Autodesk Inventor part; units mm, degrees
ref_plane "YZ Plane" through (0, 0, 0) normal (1, 0, 0) x (0, 1, 0)
ref_plane "XZ Plane" through (0, 0, 0) normal (0, 1, 0) x (-1, 0, 0)
ref_plane "XY Plane" through (0, 0, 0) normal (0, 0, 1) x (1, 0, 0)
sketch "Sketch1" plane through (0, 0, 0) normal (0, 1, 0) x (-1, 0, 0)
  line L0 (28, 0) -> (-28, 0)
  line L1 (0, -44.1) -> (0, 44.1)
  line L2 (-20, 31.5) -> (20, 31.5)
  line L3 (20, 31.5) -> (20, -31.5)
  line L4 (20, -31.5) -> (-20, -31.5)
  line L5 (-20, -31.5) -> (-20, 31.5)
  line L6 (-20, 31.5) -> (20, -31.5) construction
  line L7 (20, 31.5) -> (-20, -31.5) construction
  point P0 (0, 0)
  dimension "d0" = 40
  dimension "d1" = 63
extrude "Extrusion1" add sketch "Sketch1" along normal blind 20
sketch "Sketch2" plane through (0, 20, 0) normal (0, 1, 0) x (1, 0, 0)
  line L0 (20, 31.5) -> (-20, 31.5)
  line L1 (-20, 31.5) -> (-20, -31.5)
  line L2 (2.8, 26.5) -> (12.8, 26.5)
  line L3 (12.8, 26.5) -> (12.8, -26.5)
  line L4 (12.8, -26.5) -> (2.8, -26.5)
  line L5 (2.8, -26.5) -> (2.8, 26.5)
  line L6 (20, -31.5) -> (20, 31.5)
  dimension "d9" = 10
  dimension "d10" = 53
  dimension "d11" = 5
  dimension "d23" = 7.2
extrude "Extrusion2" cut sketch "Sketch2" against normal blind 11
sketch "Sketch3" plane through (0, 9, 0) normal (0, 1, 0) x (1, 0, 0)
  line L0 (20, -31.5) -> (20, 31.5)
  line L1 (12.8, 26.5) -> (12.8, -26.5)
  line L2 (20, 31.5) -> (-20, 31.5)
  point P0 (0, 0)
  point P1 (7.8, 14.41)
  point P2 (7.8, -14.3)
  dimension "d22" = 5
  dimension "d27" = 17.09
  dimension "d40" = 28.71
  dimension "d41" = 12.2
hole "Hole1" at (7.8, 9, -14.41) at (7.8, 9, 14.3) direction (0, -1, 0) diameter 3.242 end through all
sketch "Sketch5" plane through (0, 9, 0) normal (0, 1, 0) x (1, 0, 0)
  circle A0 centre (7.8, 14.41) radius 1.621
  line L0 (9.8207, 10.91) -> (5.7793, 10.91)
  line L1 (5.7793, 10.91) -> (3.7585, 14.41)
  line L2 (3.7585, 14.41) -> (5.7793, 17.91)
  line L3 (5.7793, 17.91) -> (9.8207, 17.91)
  line L4 (9.8207, 17.91) -> (11.8415, 14.41)
  line L5 (11.8415, 14.41) -> (9.8207, 10.91)
  line L6 (2.8, 26.5) -> (12.8, 26.5)
  line L7 (12.8, -26.5) -> (2.8, -26.5)
  circle A1 centre (7.8, -14.3) radius 1.621
  line L8 (9.8207, -17.8) -> (5.7793, -17.8)
  line L9 (5.7793, -17.8) -> (3.7585, -14.3)
  line L10 (3.7585, -14.3) -> (5.7793, -10.8)
  line L11 (5.7793, -10.8) -> (9.8207, -10.8)
  line L12 (9.8207, -10.8) -> (11.8415, -14.3)
  line L13 (11.8415, -14.3) -> (9.8207, -17.8)
  point P0 (0, 0)
  dimension "d37" = 7
  dimension "d42" = 7
extrude "Extrusion3" cut sketch "Sketch5" against normal blind 4 contours L0 L1 L2 L3 L4 L5 | A1 | L8 L9 L10 L11 L12 L13
sketch "Sketch9" plane through (-20, 0, 31.5) normal (0, 0, 1) x (1, 0, 0)
  line L0 (30.47, 20) -> (30.47, 10)
  line L1 (30.47, 10) -> (-4.63, 10)
  line L2 (-4.63, 10) -> (-4.63, 20)
  line L3 (0, 0) -> (0, 20)
  line L4 (40, 20) -> (0, 20)
  arc A0 (5.8, 20) -> (20.2, 20) centre (13, 20) ccw
  line L5 (-4.63, 20) -> (5.8, 20)
  line L6 (20.2, 20) -> (30.47, 20)
  line L7 (40, 0) -> (40, 20)
  line L8 (5.8, 20) -> (20.2, 20)
  point P0 (20, 0)
  point P1 (0, 10)
  dimension "d58" = 35.1
  dimension "d59" = 10
  dimension "d60" = 4.63
  dimension "d64" = 7.2
  dimension "d65" = 17.63
  dimension "d66" = 19.8
  dimension "d67" = 14.4
extrude "Extrusion6" add sketch "Sketch9" along normal blind 10 contours L0 L1 L3 L4 A0 | L1 L2 L5 L3
extrude "Extrusion7" cut sketch "Sketch9" against normal blind 58 contours A0 L4
sketch "Sketch10" plane through (0, 20, 0) normal (0, 1, 0) x (1, 0, 0)
  line L0 (-21.08, -37) -> (6.92, -37)
  line L1 (6.92, -37) -> (6.92, -39)
  line L2 (6.92, -39) -> (-21.08, -39)
  line L3 (-21.08, -39) -> (-21.08, -37)
  line L4 (0.2, -41.5) -> (-14.2, -41.5)
  line L5 (-24.63, -31.5) -> (-24.63, -41.5)
  point P0 (0, 0)
  dimension "d72" = 2
  dimension "d73" = 2.5
  dimension "d74" = 28
  dimension "d75" = 3.55
extrude "Extrusion8" cut sketch "Sketch10" against normal blind 8
sketch "Sketch13" plane through (0, 0, 0) normal (0, -1, 0) x (1, 0, 0)
  line L0 (-20, -31.5) -> (-20, 31.5)
  line L1 (20, -31.5) -> (-20, -31.5)
  point P0 (0, 0)
  point P1 (-7, -18.5)
  dimension "d89" = 13
  dimension "d90" = 13
ref_plane "Work Plane3" through (0, 8.8, 0) normal (0, 1, 0) x (1, 0, 0)
sketch "Sketch31" plane through (0, 8.8, 0) normal (0, 1, 0) x (1, 0, 0)
  line L0 (-4.9793, 15) -> (-9.0207, 15)
  line L1 (-9.0207, 15) -> (-11.0415, 18.5)
  line L2 (-11.0415, 18.5) -> (-9.0207, 22)
  line L3 (-9.0207, 22) -> (-4.9793, 22)
  line L4 (-4.9793, 22) -> (-2.9585, 18.5)
  line L5 (-2.9585, 18.5) -> (-4.9793, 15)
  line L6 (20, 31.5) -> (-20, 31.5)
  line L7 (-20, 31.5) -> (-20, -31.5)
  line L8 (-4.9793, -27) -> (-9.0207, -27)
  line L9 (-9.0207, -27) -> (-11.0415, -23.5)
  line L10 (-11.0415, -23.5) -> (-9.0207, -20)
  line L11 (-9.0207, -20) -> (-4.9793, -20)
  line L12 (-4.9793, -20) -> (-2.9585, -23.5)
  line L13 (-2.9585, -23.5) -> (-4.9793, -27)
  point P0 (0, 0)
  point P1 (-7, 18.5)
  point P2 (-7, -23.5)
  dimension "d159" = 13
  dimension "d160" = 13
  dimension "d161" = 7
  dimension "d171" = 7
  dimension "d172" = 13
  dimension "d173" = 42
extrude "Extrusion19" cut sketch "Sketch31" along normal through all
hole "Hole7" at (-7, 0, -18.5) direction (0, 1, 0) diameter 3.242 end through all
sketch "Sketch33" plane through (0, 8.8, 0) normal (0, 1, 0) x (1, 0, 0)
  line L0 (-20, 31.5) -> (-20, -31.5)
  line L1 (-9.0207, -20) -> (-4.9793, -20)
  point P0 (0, 0)
  point P1 (-7, -23.5001)
  dimension "d181" = 13
  dimension "d182" = 3.5001
hole "Hole8" at (-7, 8.8, 23.5001) direction (0, -1, 0) diameter 3.242 end through all
properties part number "uchwyt_strzykawka_srodek_proba_zapisania" material "PC/ABS Plastic"
For this review, take the finished solid that the model builds, in its own axes (mm). A direction names the side the tool comes from. Coordinates: 2 decimals unless noted, no trailing zeros. Order: outer loops, then holes, each group sorted by start corner. A loop starts at its lowest first (then second) coordinate and runs counter-clockwise, first axis right, second up. Notation, with made-up numbers: (26, 41.5) - (47, 41.5) arc R22 ccw to (47, 47.5) - close; hole circle Ø7 at (73, 3). An arc over 180 degrees is marked (long way). Answer as a JSON object with one key per item and string values. Group by question number.
1. For probe 1 along Z at (x, y) = (-5, 9.75); probe 2 along Z at (x, y) = (-7, 4); probe 3 along X at (y, z) = (2.1, 14.3), list the stretches that pass through material, from the lowest coordinate up.
2. We need section C-C on z = -23. State the section outline as (x, y) points, then the cut area to 3 significant figures.
3. The part is to be moulded in two halves that separate along Z. For faces 1 (the flat face through (6.92, 16, 38)), 2 (the flat face through (-7, 17, -26.5)), 3 (the flat face through (-10.045, 11.384, -20.225)), 4 (the flat face through (-20, 10, 0)), say which applies: pulls with the +Z half, pulls with the -Z half, needs draft (parallel to the pull), parting line crosses it, or undercut.
4. We need section B-B on y = 1.75. State the section outline as (x, z) points.
5. Clearance check with flat-ended pins moving along their axes: P1, Ø2, axis at x = -8, z = -17, coming from the +Y side; P2, Ø8, axis at x = -4, z = 36.5, coming from the -Y side; P3, Ø4, axis at x = -5, y = 16, coming from the +Z side; P4, Ø3, axis at x = -7, z = -18.5, coming from the +Y side. State where each tip first meets the part, or that it passes through.
6. We need section A-A on x = 7.8. State the section outline as (y, z) points.
7. We need section D-D on y = 15. State the section outline as (x, z) points.
8. For faces 5 (the cylindrical face through (-7.487, 4.338, 25.046)), 6 (the cylindrical face through (-6.84, 12.8, 40.23)), 7 (the flat face through (-10, 11.4, -16.7)), list the 3-axis set-ups (+Z, -Z, +X, -X, +Y, -Y) from which the entire face can be reached by the end or side of a thin tool; tool diameter is ignored.
Final values:
{
 "1": {"probe 1": "-31.5 to -22, -15 to 20, 27 to 31.5", "probe 2": "-31.5 to -20.12, -16.88 to 21.88, 25.12 to 31.5", "probe 3": "-20 to 6.18, 9.42 to 20"},
 "2": {"outline": "(-20, 0) - (20, 0) - (20, 20) - (12.8, 20) - (12.8, 9) - (2.8, 9) - (2.8, 20) - (0.2, 20) arc R7.2 cw to (-14.2, 20) - (-20, 20) - close", "area": "609 mm²"},
 "3": {"face 1": "undercut", "face 2": "pulls with the +Z half", "face 3": "undercut", "face 4": "needs draft"},
 "4": {"outline": "(-20, -31.5) - (20, -31.5) - (20, 31.5) - (-20, 31.5) - close; hole circle Ø3.24 at (-7, -18.5); hole circle Ø3.24 at (-7, 23.5); hole circle Ø3.24 at (7.8, -14.41); hole circle Ø3.24 at (7.8, 14.3)"},
 "5": {"P1": "y = 8.8", "P2": "y = 10", "P3": "z = -26.5", "P4": "through"},
 "6": {"outline": "(0, -31.5) - (20, -31.5) - (20, -26.5) - (9, -26.5) - (9, -17.91) - (5, -17.91) - (5, -16.03) - (0, -16.03) - close; (0, -12.79) - (5, -12.79) - (5, -10.91) - (9, -10.91) - (9, 10.8) - (5, 10.8) - (5, 12.68) - (0, 12.68) - close; (0, 15.92) - (5, 15.92) - (5, 17.8) - (9, 17.8) - (9, 26.5) - (20, 26.5) - (20, 41.5) - (10, 41.5) - (10, 31.5) - (0, 31.5) - close"},
 "7": {"outline": "(-24.63, 31.5) - (-20, 31.5) - (-20, -31.5) - (20, -31.5) - (20, 31.5) - (10.47, 31.5) - (10.47, 41.5) - (-1.82, 41.5) - (-1.82, 39) - (6.92, 39) - (6.92, 37) - (-1.82, 37) - (-1.82, -26.5) - (-12.18, -26.5) - (-12.18, 37) - (-21.08, 37) - (-21.08, 39) - (-12.18, 39) - (-12.18, 41.5) - (-24.63, 41.5) - close; hole (2.8, -26.5) - (12.8, -26.5) - (12.8, 26.5) - (2.8, 26.5) - close"},
 "8": {"face 5": "+Y, -Y", "face 6": "+Z, +Y", "face 7": "+Y"}
}
